from build123d import *

# Parameters (mm, degrees)
SKETCH1_W           = 4
SKETCH1_H           = 1.5
BOSS_EXTRUDE1_DEPTH = 3
SKETCH4_W           = 15
SKETCH4_H           = 3
CUT_EXTRUDE3_DEPTH  = 158.575378787
SKETCH7_R           = 1.5
CUT_EXTRUDE6_DEPTH  = 10


with BuildPart() as part:
    # Sketch1 → Boss-Extrude1 (new body)
    with BuildSketch(Plane(origin=(0, 0, 0), x_dir=(1, 0, 0), z_dir=(0, 1, 0))):
        Polygon((0, 90), (0, 130), (20, 130), (20, 90), (89, 90), (89, 0), (0, 0), align=None)
        with Locations((10, 125.75)):
            Rectangle(SKETCH1_W, SKETCH1_H, mode=Mode.SUBTRACT)
    extrude(amount=BOSS_EXTRUDE1_DEPTH)

    # Sketch4 → Cut-Extrude3 (cut, through all)
    with BuildSketch(Plane.XY):
        with Locations((81.5, 1.5)):
            Rectangle(SKETCH4_W, SKETCH4_H)
    extrude(amount=-CUT_EXTRUDE3_DEPTH, mode=Mode.SUBTRACT)

    # Sketch7 → Cut-Extrude6 (cut)
    with BuildSketch(Plane(origin=(0, 3, 0), x_dir=(1, 0, 0), z_dir=(0, 1, 0))):
        with Locations(Location((39, 83.5, 0), (0, 0, 270))):
            Circle(SKETCH7_R)
        with Locations(Location((55, 83.5, 0), (0, 0, 270))):
            Circle(SKETCH7_R)
    extrude(amount=-CUT_EXTRUDE6_DEPTH, mode=Mode.SUBTRACT)


solid = part.part
The model under review builds one solid part; all positions refer to its coordinate system, in mm. A direction names the side the tool comes from. Coordinates: 2 decimals unless noted, no trailing zeros. Write each loop counter-clockwise with the first axis right and the second up, starting at its lowest first coordinate (ties: lowest second). Pieces come first, ordered by that corner, then holes. Notation, with made-up numbers: (50, -17.5) - (77, -17.5) arc R14 ccw to (77, -1.5) - close; hole circle Ø5 at (68, 77.25). An arc over 180 degrees is marked (long way). Answer as a JSON object with one key per item and string values. Group by question number.
1. Add section D-D (x = 61.5). Give the boundary of the cut face in (y, z).
2. Clearance check with flat-ended pins moving along their axes: pin 1 Ø1.8 at (x, z) = (39, -83.5) entering from -Y; pin 2 Ø1.2 at (y, z) = (1.5, -125.5) entering from +X. State where each tip first meets the part, or that it passes through.
3. Add section C-C (z = -83.5). Give the boundary of the cut face in (x, y), plus the area to 3 significant figures.
4. Add section B-B (x = 39). Give the boundary of the cut face in (y, z), plus the area to 3 significant figures.
5. Machinability: for faces 1 (the face through (10, 1, -126.5)), 2 (the face through (38, 3, -51)), 3 (the face through (47, 1, -90)), which of the approach directions +Z, -Z, +X, -X, +Y, -Y give a long, thin tool a straight path to every point of the face, cutting with its end or side? Answer none if there is none.
6. To check wall thickness, follow probe 1 along X at (y, z) = (1.7, -83.5); probe 2 along X at (y, z) = (1.75, -84); probe 3 along X at (y, z) = (1.85, -122). State the ranges of each line that lie inside material, in increasing order.
7. Mouldability with a two-part tool opening along X and no side actions: class faces 4 (the face through (38, 1, 0)), 5 (the face through (55, 2, -82)), 6 (the face through (20, 1, -110)) as pulls with the +X half, pulls with the -X half, needs draft (parallel to the pull), parting line crosses it, or undercut.
8. Add section A-A (y = 1.55). Give the boundary of the cut face in (x, z).
Findings:
{
 "1": {"outline": "(0, -90) - (3, -90) - (3, 0) - (0, 0) - close"},
 "2": {"pin 1": "through", "pin 2": "x = 20"},
 "3": {"outline": "(0, 0) - (37.5, 0) - (37.5, 3) - (0, 3) - close; (40.5, 0) - (53.5, 0) - (53.5, 3) - (40.5, 3) - close; (56.5, 0) - (74, 0) - (74, 3) - (56.5, 3) - close", "area": "204 mm²"},
 "4": {"outline": "(0, -90) - (3, -90) - (3, -85) - (0, -85) - close; (0, -82) - (3, -82) - (3, 0) - (0, 0) - close", "area": "261 mm²"},
 "5": {"face 1": "+Y, -Y", "face 2": "+Z, -Z, +X, -X, +Y", "face 3": "-Z, +X, +Y, -Y"},
 "6": {"probe 1": "0 to 37.5, 40.5 to 53.5, 56.5 to 74", "probe 2": "0 to 37.59, 40.41 to 53.59, 56.41 to 74", "probe 3": "0 to 20"},
 "7": {"face 4": "needs draft", "face 5": "undercut", "face 6": "pulls with the +X half"},
 "8": {"outline": "(0, -130) - (20, -130) - (20, -90) - (74, -90) - (74, 0) - (0, 0) - close; hole (8, -126.5) - (12, -126.5) - (12, -125) - (8, -125) - close; hole circle Ø3 at (39, -83.5); hole circle Ø3 at (55, -83.5)"}
}
